Could you check a few things on this model? Use its own coordinates, in mm. A direction names the side the tool comes from. Give positions to 0.01 mm unless a question says otherwise; leave off trailing zeros. Order: outer loops, then holes, each group sorted by start corner. A loop starts at its lowest first (then second) coordinate and runs counter-clockwise, first axis right, second up. Notation, with made-up numbers: M 71,-4 L 91,-4 A11 ccw 91,9 Z; hole C 45.5,50.5 d10. An arc over 180 degrees is marked long. Answer in a Markdown table with one row per item. Add a question column.
```python
from build123d import *

# Parameters (mm, degrees)
SKETCH1_W           = 39
SKETCH1_H           = 57
BOSS_EXTRUDE1_DEPTH = 6
SKETCH2_R           = 4.75
SKETCH2_R_2         = 1.75
BOSS_EXTRUDE2_DEPTH = 6
FILLET4_R           = 10
SKETCH4_W           = 10.304705379
SKETCH4_H           = 12
BOSS_EXTRUDE3_DEPTH = 6
FILLET5_R           = 10
CUT_EXTRUDE2_DEPTH  = 3.5
FILLET7_R           = 2
FILLET8_R           = 2
FILLET9_R           = 2


with BuildPart() as part:
    # Sketch1 → Boss-Extrude1 (new body)
    with BuildSketch(Plane.XY):
        Rectangle(SKETCH1_W, SKETCH1_H)
    extrude(amount=BOSS_EXTRUDE1_DEPTH)

    # Sketch2 → Boss-Extrude2 (add)
    # profile 1 of 4: a face of its own
    with BuildSketch(Plane.XY.offset(6)):
        with BuildLine():
            ThreePointArc((33.5, 17.75), (28.75, 22.5), (33.5, 27.25))
            Line((33.5, 27.25), (19.5, 27.25))
            Line((19.5, 27.25), (19.5, 17.75))
            Line((19.5, 17.75), (33.5, 17.75))
        make_face()
    # profile 2 of 4: a face of its own
    with BuildSketch(Plane.XY.offset(6)):
        with BuildLine():
            Line((-19.5, -6.75), (-29.5, -6.75))
            ThreePointArc((-29.5, -6.75), (-26.141242789, -8.141242789), (-24.75, -11.5))
            ThreePointArc((-24.75, -11.5), (-26.141242789, -14.858757211), (-29.5, -16.25))
            Line((-29.5, -16.25), (-19.5, -16.25))
            Line((-19.5, -16.25), (-19.5, -6.75))
        make_face()
    # profile 3 of 4: a face of its own
    with BuildSketch(Plane.XY.offset(6)):
        with Locations((-29.5, -11.5)):
            Circle(SKETCH2_R)
        with Locations((-29.5, -11.5)):
            Circle(SKETCH2_R_2, mode=Mode.SUBTRACT)
    # profile 4 of 4: a face of its own
    with BuildSketch(Plane.XY.offset(6)):
        with Locations((33.5, 22.5)):
            Circle(SKETCH2_R)
        with Locations((33.5, 22.5)):
            Circle(SKETCH2_R_2, mode=Mode.SUBTRACT)
    extrude(amount=-BOSS_EXTRUDE2_DEPTH)

    # Fillet4
    fillet4_edges = [part.edges().sort_by_distance(p)[0] for p in [
        (-19.5, 28.5, 3),
        (19.5, -28.5, 3),
    ]]
    fillet(fillet4_edges, radius=FILLET4_R)

    # Sketch4 → Boss-Extrude3 (add)
    with BuildSketch(Plane.XY.offset(6)):
        with Locations((24.652352689, 22.5)):
            Rectangle(SKETCH4_W, SKETCH4_H)
    extrude(amount=-BOSS_EXTRUDE3_DEPTH)

    # Fillet5
    # the kernel refuses this fillet: 10 mm, written as the material it adds along each edge
    with BuildSketch(Plane(origin=(29.804705379, 17.75, 6), x_dir=(0, -1, 0), z_dir=(0, 0, -1))) as fillet5_piece_1:
        with BuildLine():
            CenterArc((9.947871925, -4.934270359), FILLET5_R, 150.433919307, 24.747651836)
            Line((-0.016787007, -4.094286808), (-1.0132529, -4.010288453))
            ThreePointArc((-1.0132529, -4.010288453), (-1, -3.695294621), (-1, 0))
            Line((-1, 0), (0, 1))
            ThreePointArc((0, 1), (0.625, 1), (0.380212808, 0.493427036))
            Line((0.380212808, 0.493427036), (1.25, 0))
        make_face()
    extrude(amount=6)
    with BuildSketch(Plane(origin=(29.804705379, 27.25, 0), x_dir=(0.9999915946740242, -0.004100070889875189, 0), z_dir=(0, 0, 1))) as fillet5_piece_2:
        with BuildLine():
            CenterArc((4.893441905, 9.968019168), FILLET5_R, 240.668836723, 24.747651836)
            Line((-0.005125089, 1.249989493), (-0.494981788, 0.378186526))
            ThreePointArc((-0.494981788, 0.378186526), (-1.002554139, 0.620894676), (-0.999991595, -0.004100071))
            Line((-0.999991595, -0.004100071), (0.004100071, -0.999991595))
            ThreePointArc((0.004100071, -0.999991595), (3.699363631, -0.984840625), (4.014409153, -0.996801917))
            Line((4.014409153, -0.996801917), (4.094321222, 0))
        make_face()
    extrude(amount=6)
    with BuildSketch(Plane(origin=(19.5, 16.5, 6), x_dir=(0, -1, 0), z_dir=(0, 0, -1)), Plane(origin=(-19.5, -6.75, 6), x_dir=(0, 1, 0), z_dir=(0, 0, -1)), Plane(origin=(-19.5, -16.25, 6), x_dir=(-1, 0, 0), z_dir=(0, 0, -1))) as fillet5_piece_3:
        with BuildLine():
            CenterArc((FILLET5_R, -FILLET5_R), FILLET5_R, 90, 90)
            Line((0, -FILLET5_R), (-FILLET5_R * 0.02, -FILLET5_R))
            Line((-FILLET5_R * 0.02, -FILLET5_R), (-FILLET5_R * 0.02, FILLET5_R * 0.02))
            Line((-FILLET5_R * 0.02, FILLET5_R * 0.02), (FILLET5_R, FILLET5_R * 0.02))
            Line((FILLET5_R, FILLET5_R * 0.02), (FILLET5_R, 0))
        make_face()
    extrude(amount=6)

    # Sketch5 → Cut-Extrude2 (cut)
    with BuildSketch(Plane(origin=(0, 0, 0), x_dir=(-1, 0, 0), z_dir=(0, 0, -1))):
        with BuildLine():
            Line((16.5, 3.25), (16.5, 18.5))
            ThreePointArc((16.5, 18.5), (14.449747468, 23.449747468), (9.5, 25.5))
            Line((9.5, 25.5), (-20.150604469, 25.5))
            Line((-20.150604469, 25.5), (-20.150604469, 15.532652058))
            ThreePointArc((-20.150604469, 15.532652058), (-17.447155068, 11.371234859), (-16.5, 6.5))
            Line((-16.5, 6.5), (-16.5, -18.5))
            ThreePointArc((-16.5, -18.5), (-14.449747468, -23.449747468), (-9.5, -25.5))
            Line((-9.5, -25.5), (16.521652648, -25.5))
            ThreePointArc((16.521652648, -25.5), (17.716131688, -20.759968343), (20.576715851, -16.796164799))
            Line((20.576715851, -16.796164799), (20.307611845, -5.942388155))
            ThreePointArc((20.307611845, -5.942388155), (17.489566077, -1.724884621), (16.5, 3.25))
        make_face()
    extrude(amount=-CUT_EXTRUDE2_DEPTH, mode=Mode.SUBTRACT)

    # Fillet7
    fillet7_edges = [part.edges().sort_by_distance(p)[0] for p in [
        (-19.5, -28.5, 3),
    ]]
    fillet(fillet7_edges, radius=FILLET7_R)

    # Fillet8
    # the kernel refuses this fillet: 2 mm, written as the material it takes off along each edge
    with BuildSketch(Plane(origin=(34.738975739, 7.802128075, 6), x_dir=(-0.8500291529283407, 0.5267356444858536, 0), z_dir=(-0.5267356444858536, -0.8500291529283407, 0))) as fillet8_piece_1:
        with BuildLine():
            CenterArc((10 + FILLET8_R, FILLET8_R), FILLET8_R, 180, 90)
            Line((10, FILLET8_R), (10, 0))
            Line((10, 0), (10 + FILLET8_R, 0))
        make_face()
    revolve(axis=Axis((34.738975739, 7.802128075, 6), (0, 0, -1)), revolution_arc=53.396411501, mode=Mode.SUBTRACT)
    with BuildSketch(Plane(origin=(34.738975739, 37.197871925, 6), x_dir=(-0.8500291529284019, -0.5267356444857548, 0), z_dir=(-0.5267356444857548, 0.8500291529284019, 0))) as fillet8_piece_2:
        with BuildLine():
            CenterArc((10 + FILLET8_R, -FILLET8_R), FILLET8_R, 90, 90)
            Line((10, -FILLET8_R), (10, 0))
            Line((10, 0), (10 + FILLET8_R, 0))
        make_face()
    revolve(axis=Axis((34.738975739, 37.197871925, 6), (0, 0, 1)), revolution_arc=53.396411501, mode=Mode.SUBTRACT)
    with BuildSketch(Plane(origin=(29.5, 6.5, 6), x_dir=(-1, 0, 0), z_dir=(0, -1, 0))) as fillet8_piece_3:
        with BuildLine():
            CenterArc((10 + FILLET8_R, FILLET8_R), FILLET8_R, 180, 90)
            Line((10, FILLET8_R), (10, 0))
            Line((10, 0), (10 + FILLET8_R, 0))
        make_face()
    revolve(axis=Axis((29.5, 6.5, 6), (0, 0, -1)), revolution_arc=90, mode=Mode.SUBTRACT)
    with BuildSketch(Plane(origin=(19.5, -18.5, 6), x_dir=(-1, 0, 0), z_dir=(0, 1, 0))) as fillet8_piece_4:
        with BuildLine():
            CenterArc((FILLET8_R, -FILLET8_R), FILLET8_R, 90, 90)
            Line((0, -FILLET8_R), (0, 0))
            Line((0, 0), (FILLET8_R, 0))
        make_face()
    extrude(amount=25, mode=Mode.SUBTRACT)
    with BuildSketch(Plane(origin=(9.5, -18.5, 6), x_dir=(0, -1, 0), z_dir=(-1, 0, 0))) as fillet8_piece_5:
        with BuildLine():
            CenterArc((10 - FILLET8_R, -FILLET8_R), FILLET8_R, 0, 90)
            Line((10, -FILLET8_R), (10, 0))
            Line((10, 0), (10 - FILLET8_R, 0))
        make_face()
    revolve(axis=Axis((9.5, -18.5, 6), (0, 0, 1)), revolution_arc=90, mode=Mode.SUBTRACT)
    with BuildSketch(Plane(origin=(-17.5, -28.5, 6), x_dir=(0, 1, 0), z_dir=(1, 0, 0))) as fillet8_piece_6:
        with BuildLine():
            CenterArc((FILLET8_R, -FILLET8_R), FILLET8_R, 90, 90)
            Line((0, -FILLET8_R), (0, 0))
            Line((0, 0), (FILLET8_R, 0))
        make_face()
    extrude(amount=27, mode=Mode.SUBTRACT)
    with BuildSketch(Plane(origin=(-17.5, -26.5, 6), x_dir=(-1, 0, 0), z_dir=(0, 1, 0))) as fillet8_piece_7:
        with BuildLine():
            CenterArc((2 - FILLET8_R, -FILLET8_R), FILLET8_R, 0, 90)
            Line((2, -FILLET8_R), (2, 0))
            Line((2, 0), (2 - FILLET8_R, 0))
        make_face()
    revolve(axis=Axis((-17.5, -26.5, 6), (0, 0, 1)), revolution_arc=90, mode=Mode.SUBTRACT)
    with BuildSketch(Plane(origin=(-19.5, -26.25, 6), x_dir=(1, 0, 0), z_dir=(0, -1, 0))) as fillet8_piece_8:
        with BuildLine():
            CenterArc((FILLET8_R, -FILLET8_R), FILLET8_R, 90, 90)
            Line((0, -FILLET8_R), (0, 0))
            Line((0, 0), (FILLET8_R, 0))
        make_face()
    extrude(amount=0.25, mode=Mode.SUBTRACT)
    with BuildSketch(Plane(origin=(-29.5, -26.25, 6), x_dir=(0, 1, 0), z_dir=(-1, 0, 0))) as fillet8_piece_9:
        with BuildLine():
            CenterArc((10 + FILLET8_R, FILLET8_R), FILLET8_R, 180, 90)
            Line((10, FILLET8_R), (10, 0))
            Line((10, 0), (10 + FILLET8_R, 0))
        make_face()
    revolve(axis=Axis((-29.5, -26.25, 6), (0, 0, -1)), revolution_arc=90, mode=Mode.SUBTRACT)
    with BuildSketch(Plane(origin=(-29.5, -11.5, 6), x_dir=(0, 1, 0), z_dir=(1, 0, 0))) as fillet8_piece_10:
        with BuildLine():
            CenterArc((4.75 - FILLET8_R, -FILLET8_R), FILLET8_R, 0, 90)
            Line((4.75, -FILLET8_R), (4.75, 0))
            Line((4.75, 0), (4.75 - FILLET8_R, 0))
        make_face()
    revolve(axis=Axis((-29.5, -11.5, 6), (0, 0, 1)), revolution_arc=180, mode=Mode.SUBTRACT)
    with BuildSketch(Plane(origin=(-29.5, 3.25, 6), x_dir=(1, 0, 0), z_dir=(0, 1, 0))) as fillet8_piece_11:
        with BuildLine():
            CenterArc((10 + FILLET8_R, FILLET8_R), FILLET8_R, 180, 90)
            Line((10, FILLET8_R), (10, 0))
            Line((10, 0), (10 + FILLET8_R, 0))
        make_face()
    revolve(axis=Axis((-29.5, 3.25, 6), (0, 0, -1)), revolution_arc=90, mode=Mode.SUBTRACT)
    with BuildSketch(Plane(origin=(-19.5, 18.5, 6), x_dir=(1, 0, 0), z_dir=(0, -1, 0))) as fillet8_piece_12:
        with BuildLine():
            CenterArc((FILLET8_R, -FILLET8_R), FILLET8_R, 90, 90)
            Line((0, -FILLET8_R), (0, 0))
            Line((0, 0), (FILLET8_R, 0))
        make_face()
    extrude(amount=15.25, mode=Mode.SUBTRACT)
    with BuildSketch(Plane(origin=(-9.5, 18.5, 6), x_dir=(0, 1, 0), z_dir=(1, 0, 0))) as fillet8_piece_13:
        with BuildLine():
            CenterArc((10 - FILLET8_R, -FILLET8_R), FILLET8_R, 0, 90)
            Line((10, -FILLET8_R), (10, 0))
            Line((10, 0), (10 - FILLET8_R, 0))
        make_face()
    revolve(axis=Axis((-9.5, 18.5, 6), (0, 0, 1)), revolution_arc=90, mode=Mode.SUBTRACT)
    with BuildSketch(Plane(origin=(33.5, 22.5, 6), x_dir=(0.08399835516458835, 0.9964658932094184, 0), z_dir=(-0.9964658932094184, 0.08399835516458835, 0))) as fillet8_piece_14:
        with BuildLine():
            CenterArc((4.75 - FILLET8_R, FILLET8_R), FILLET8_R, 270, 90)
            Line((4.75, FILLET8_R), (4.75, 0))
            Line((4.75, 0), (4.75 - FILLET8_R, 0))
        make_face()
    revolve(axis=Axis((33.5, 22.5, 6), (0, 0, -1)), revolution_arc=170.363142288, mode=Mode.SUBTRACT)
    with BuildSketch(Plane(origin=(-9.5, 28.5, 6), x_dir=(0, -1, 0), z_dir=(1, 0, 0))) as fillet8_piece_15:
        with BuildLine():
            CenterArc((FILLET8_R, FILLET8_R), FILLET8_R, 180, 90)
            Line((0, FILLET8_R), (0, 0))
            Line((0, 0), (FILLET8_R, 0))
        make_face()
    extrude(amount=44.304705379, mode=Mode.SUBTRACT)
    with BuildSketch(Plane(origin=(34.804705379, 16.5, 6), x_dir=(0, 1, 0), z_dir=(-1, 0, 0))) as fillet8_piece_16:
        with BuildLine():
            CenterArc((FILLET8_R, FILLET8_R), FILLET8_R, 180, 90)
            Line((0, FILLET8_R), (0, 0))
            Line((0, 0), (FILLET8_R, 0))
        make_face()
    extrude(amount=5.304705379, mode=Mode.SUBTRACT)

    # Fillet9
    fillet9_edges = [part.edges().sort_by_distance(p)[0] for p in [
        (-16.5, 10.875, 3.5),
        (-3.510826324, -25.5, 3.5),
        (14.449747468, -23.449747468, 3.5),
        (16.5, -6, 3.5),
        (5.325302234, 25.5, 3.5),
        (-14.449747468, 23.449747468, 3.5),
        (-17.489566077, -1.724884621, 3.5),
        (-20.442163848, -11.369276477, 3.5),
        (-17.716131688, -20.759968343, 3.5),
        (17.447155068, 11.371234859, 3.5),
        (20.150604469, 20.516326029, 3.5),
    ]]
    fillet(fillet9_edges, radius=FILLET9_R)


solid = part.part
```
1. Will these pins go through, and if not, where does the flat tip stop? P1, Ø1.2, axis at y = 21.5, z = 1, coming from the -X side; P2, Ø2, axis at x = -29.5, y = -11.5, coming from the -Z side; P3, Ø3, axis at y = 8, z = 2, coming from the +X side; P4, Ø1.2, axis at y = 8.5, z = 0.5, coming from the +X side.
2. For faces 1 (the cylindrical face through (16.65, -25.49, 2.03)), 2 (the cylindrical face through (-18.9, 10.98, 5.43)), 3 (the cylindrical face through (17.474, 11.436, 0.74)), which set-ups out of +Z, -Z, +X, -X, +Y, -Y let a thin tool reach every point of the face, with its end or its side?
3. Suppose I cut it at A-A on x = 6.5. List the corners of the cut face in (y, z) for me, plus the area to 4 significant figures.
4. If I drill on line 1 along X through (y, z) = (23, 0.5); line 2 along Y through (x, z) = (-29.5, 4.1); line 3 along Z through (x, y) = (13, -9), over which ranges is the centre line in solid material (lowest first)? Write a range as [from, to].
5. Suppose I cut it at B-B on z = 4.75. List the corners of the cut face in (x, y) for me, plus the area to 3 significant figures.
6. Thinking about a two-plate mould opening in Y: for faces 4 (the cylindrical face through (-14.5, 23.4, 0.7)), 5 (the flat face through (19.5, -6, 2)), 6 (the flat face through (20.151, 21, 1)), 7 (the cylindrical face through (-18.93, -27.9, 2.03)), which applies, pulls with the +Y half, pulls with the -Y half, needs draft (parallel to the pull), parting line crosses it, or undercut?
Findings below:
| question | item | result |
|---|---|---|
| 1 | P1 | x = -19.21 |
| 1 | P2 | through |
| 1 | P3 | x = 19.96 |
| 1 | P4 | x = 19.84 |
| 2 | face 1 | +Z, -Z, +X, -Y |
| 2 | face 2 | +Z, -X, +Y |
| 2 | face 3 | -Z |
| 3 | outline | M -28.5,0 L -25.5,0 L -25.5,1.5 A2 cw -23.5,3.5 L 23.5,3.5 A2 cw 25.5,1.5 L 25.5,0 L 28.5,0 L 28.5,4 A2 ccw 26.5,6 L -26.5,6 A2 ccw -28.5,4 Z |
| 3 | area | 163.5 mm2 |
| 4 | line 1 | [-18.43, -14.86], [20.15, 31.82], [35.18, 38.22] |
| 4 | line 2 | [-16.25, -13.25], [-9.75, -6.75] |
| 4 | line 3 | [3.5, 6] |
| 5 | outline | M -29.5,-16.1 A10.15 cw -19.35,-26.25 L -19.35,-26.5 A1.85 ccw -17.5,-28.35 L 9.5,-28.35 A9.85 ccw 19.35,-18.5 L 19.35,6.5 A10.15 cw 29.5,16.65 L 29.77,16.65 A10.15 cw 33.89,17.91 A4.6 ccw 33.89,27.09 A10.15 cw 29.77,28.35 L -9.5,28.35 A9.85 ccw -19.35,18.5 L -19.35,3.25 A10.15 cw -29.5,-6.9 A4.6 ccw Z; hole C -29.5,-11.5 d3.5; hole C 33.5,22.5 d3.5 |
| 5 | area | 2,520 mm2 |
| 6 | face 4 | undercut |
| 6 | face 5 | needs draft |
| 6 | face 6 | undercut |
| 6 | face 7 | pulls with the -Y half |
